Geometry: final body of the model. Coordinates: model frame, mm. A direction names the side the tool comes from. Give positions to 0.01 mm unless a question says otherwise; leave off trailing zeros. Write each loop counter-clockwise with the first axis right and the second up, starting at its lowest first coordinate (ties: lowest second). Pieces come first, ordered by that corner, then holes. Notation, with made-up numbers: (1.25, 21) -> (8.25, 21) arc R19 ccw to (8.25, 51) -> close; hole circle Ø3 at (-23, 18). An arc over 180 degrees is marked (long way). Answer in a Markdown table with one row per item. Add a question column.
from build123d import *

# Parameters (mm, degrees)
F0_W      = 50
F0_H      = 50
F1_DEPTH  = 8.6
F2_W      = 45
F2_H      = 45
F3_DEPTH  = 1.6
F3_TAPER  = 3
F5_DEPTH  = 4.5
F5_TAPER  = 3
F6_R      = 3
F7_DEPTH  = 7
F8_R      = 0.5
F9_R      = 1.5095
F10_DEPTH = 5
F11_R     = 2


with BuildPart() as f1:
    # F0 (on Top) → F1 (new body)
    with BuildSketch(Plane.XY):
        Rectangle(F0_W, F0_H)
    extrude(amount=-F1_DEPTH)

    # F2 (on face) → F3 (cut)
    with BuildSketch(Plane.XY):
        Rectangle(F2_W, F2_H)
    extrude(amount=-F3_DEPTH, taper=F3_TAPER, mode=Mode.SUBTRACT)

    # F4 (on face) → F5 (cut)
    with BuildSketch(Plane.XY.offset(-1.6)):
        with BuildLine():
            Line((13.5, 18.5), (13.5, 20.9161475531))
            Line((13.5, 20.9161475531), (5, 20.9161475531))
            Line((5, 20.9161475531), (5, 17.5))
            ThreePointArc((5, 17.5), (0, 12.5), (-5, 17.5))
            Line((-5, 17.5), (-5, 20.9161475531))
            Line((-5, 20.9161475531), (-20.9161475531, 20.9161475531))
            Line((-20.9161475531, 20.9161475531), (-20.9161475531, -13.5))
            Line((-20.9161475531, -13.5), (-18.5, -13.5))
            ThreePointArc((-18.5, -13.5), (-14.9644660941, -14.9644660941), (-13.5, -18.5))
            Line((-13.5, -18.5), (-13.5, -20.9161475531))
            Line((-13.5, -20.9161475531), (-5, -20.9161475531))
            Line((-5, -20.9161475531), (-5, -17.5))
            ThreePointArc((-5, -17.5), (0, -12.5), (5, -17.5))
            Line((5, -17.5), (5, -20.9161475531))
            Line((5, -20.9161475531), (20.9161475531, -20.9161475531))
            Line((20.9161475531, -20.9161475531), (20.9161475531, 13.5))
            Line((20.9161475531, 13.5), (18.5, 13.5))
            ThreePointArc((18.5, 13.5), (14.9644660941, 14.9644660941), (13.5, 18.5))
        make_face()
    extrude(amount=-F5_DEPTH, taper=F5_TAPER, mode=Mode.SUBTRACT)

    # F6 (on face) → F7 (cut, through all)
    with BuildSketch(Plane.XY.offset(-1.6)):
        with Locations((18.5, 18.5)):
            Circle(F6_R)
        with Locations((-18.5, -18.5)):
            Circle(F6_R)
    extrude(amount=-F7_DEPTH, mode=Mode.SUBTRACT)

    # F8
    f8_edges = [f1.edges().sort_by_distance(p)[0] for p in [
        (0, -25, -8.6),
        (-25, -25, -4.3),
        (-25, 0, -8.6),
        (-21.5, -18.5, -8.6),
        (15.5, 18.5, -8.6),
        (-25, 25, -4.3),
        (0, 25, -8.6),
        (25, 25, -4.3),
        (25, 0, -8.6),
        (25, -25, -4.3),
    ]]
    fillet(f8_edges, radius=F8_R)

    # F9 (on face) → F10 (cut)
    with BuildSketch(Plane.XY.offset(-1.6)):
        with Locations((0, 17.5)):
            Circle(F9_R)
        with Locations((0, -17.5)):
            Circle(F9_R)
    extrude(amount=-F10_DEPTH, mode=Mode.SUBTRACT)

    # F11
    f11_edges = [f1.edges().sort_by_distance(p)[0] for p in [
        (5.117918, 20.79823, -3.85),
        (0, 12.264165, -6.1),
        (-5.117918, 20.79823, -3.85),
        (-5.117918, -20.79823, -3.85),
        (-5.235835, -19.090156, -6.1),
        (5.117918, -20.79823, -3.85),
    ]]
    fillet(f11_edges, radius=F11_R)


solid = f1.part
Q1. Line query: probe 1 along X at (y, z) = (-4.5, -1.5); probe 2 along Y at (x, z) = (0, -4.4); probe 3 along Y at (x, z) = (-19, -3.75). Output: solid intervals per line, ascending. Write a range as from..to.
Q2. Access query for faces 4 (the flat face through (0, 18, -6.6)), 5 (the flat face through (0, 25, -4)). Directions: +Z, -Z, +X, -X, +Y, -Y. A direction counts if a zero-diameter tool reaches every point of the face in a straight line with its end or side. Return the directions, or none.
Q3. Section A-A on z = -7.5. Return loops of the section in (x, y).
Q4. Section B-B on z = -5. Count the separate pieces of the cut face and the enclosed holes in it, and give its area (3 significant figures).
Q5. Pull-direction query (Y, two-part tool) for faces 1 (the flat face through (0, -13, -1.6)), 2 (the flat face through (25, 0, -4)), 3 (the flat face through (0, -25, -4)); classes: +Y half, -Y half, draft (parallel to the pull), parting line (faces both ways), or undercut.
Q6. Contact query for flat-ended pins moving along their axis: pin 1 Ø0.9 at (x, y) = (-0.5, -17) entering from +Z; pin 2 Ø3.5 at (x, y) = (0, 17.5) entering from +Z; pin 3 Ø6 at (x, y) = (-13, -20) entering from +Z; pin 4 Ø5 at (x, y) = (18.5, 18.5) entering from -Z. Output: stop coordinate, or through.
Checks:
| question | item | result |
|---|---|---|
| 1 | probe 1 | -25..-22.42, 22.42..25 |
| 1 | probe 2 | -25..-19.01, -15.99..-12.34, 12.34..15.99, 19.01..25 |
| 1 | probe 3 | -25..-21.46, -15.54..-13.39, 20.8..25 |
| 2 | face 4 | +Z |
| 2 | face 5 | +Z, -Z, +X, -X, +Y |
| 3 | outline | (-25, -24.5) arc R0.5 ccw to (-24.5, -25) -> (24.5, -25) arc R0.5 ccw to (25, -24.5) -> (25, 24.5) arc R0.5 ccw to (24.5, 25) -> (-24.5, 25) arc R0.5 ccw to (-25, 24.5) -> close; hole circle Ø6 at (-18.5, -18.5); hole circle Ø6 at (18.5, 18.5) |
| 4 | separate pieces | 1 |
| 4 | enclosed holes | 5 |
| 4 | area | 969 mm^2 |
| 5 | face 1 | undercut |
| 5 | face 2 | draft |
| 5 | face 3 | -Y half |
| 6 | pin 1 | z = -6.6 |
| 6 | pin 2 | z = -1.6 |
| 6 | pin 3 | z = 0 |
| 6 | pin 4 | through |
